```python
from build123d import *

# Parameters (mm, degrees)
SKETCH_1_W          = 58.5
SKETCH_1_H          = 42
EXTRUDE_1_DEPTH     = 123
CUT_EXTRUDE_1_DEPTH = 120
SKETCH_3_W          = 52.5
SKETCH_3_H          = 3
CUT_EXTRUDE_2_DEPTH = 25
FILLET_1_R          = 3
SKETCH_4_W          = 7
SKETCH_4_H          = 123
EXTRUDE_2_DEPTH     = 3
HOLE_WIZARD_1_D     = 3.5
SKETCH_7_2_W        = 7
SKETCH_7_2_H        = 83
CUT_EXTRUDE_3_DEPTH = 3
SKETCH_9_W          = 52.5
SKETCH_9_H          = 36
EXTRUDE_3_DEPTH     = 10


with BuildPart() as part:
    # 草图1 → 凸台-拉伸1 (new body)
    with BuildSketch(Plane(origin=(0, 0, 0), x_dir=(1, 0, 0), z_dir=(0, 1, 0))):
        with Locations((29.25, 21)):
            Rectangle(SKETCH_1_W, SKETCH_1_H)
    extrude(amount=EXTRUDE_1_DEPTH)

    # 草图2 → 切除-拉伸1 (cut)
    with BuildSketch(Plane(origin=(0, 123, 0), x_dir=(1, 0, 0), z_dir=(0, 1, 0))):
        Polygon((3, 3), (4.178571429, 3), (54.321428571, 39), (3, 39), align=None)
        Polygon((54.321428571, 39), (4.178571429, 3), (55.5, 3), (55.5, 39), align=None)
    extrude(amount=-CUT_EXTRUDE_1_DEPTH, mode=Mode.SUBTRACT)

    # 草图3 → 切除-拉伸2 (cut)
    with BuildSketch(Plane(origin=(0, 123, 0), x_dir=(1, 0, 0), z_dir=(0, 1, 0))):
        with Locations((29.25, 1.5)):
            Rectangle(SKETCH_3_W, SKETCH_3_H)
    extrude(amount=-CUT_EXTRUDE_2_DEPTH, mode=Mode.SUBTRACT)

    # 圆角1
    fillet_1_edges = [part.edges().sort_by_distance(p)[0] for p in [
        (3, 98, -1.5),
        (55.5, 98, -1.5),
    ]]
    fillet(fillet_1_edges, radius=FILLET_1_R)

    # 草图4 → 凸台-拉伸2 (add)
    with BuildSketch(Plane(origin=(0, 0, -42), x_dir=(-1, 0, 0), z_dir=(0, 0, -1))):
        with Locations((-62, 61.5)):
            Rectangle(SKETCH_4_W, SKETCH_4_H)
        with Locations((3.5, 61.5)):
            Rectangle(SKETCH_4_W, SKETCH_4_H)
    extrude(amount=-EXTRUDE_2_DEPTH)

    # 孔1 (through all)
    with Locations(Plane(origin=(0, 0, -42), x_dir=(-1, 0, 0), z_dir=(0, 0, -1))):
        with Locations((-62, 3.5), (3.5, 3.5), (3.5, 119.5), (-62, 119.5)):
            Hole(HOLE_WIZARD_1_D / 2)

    # Sketch 7 2 → 切除-拉伸3 (cut)
    with BuildSketch(Plane(origin=(0, 0, -42), x_dir=(-1, 0, 0), z_dir=(0, 0, -1))):
        with Locations((3.5, 61.5)):
            Rectangle(SKETCH_7_2_W, SKETCH_7_2_H)
        with Locations((-62, 61.5)):
            Rectangle(SKETCH_7_2_W, SKETCH_7_2_H)
    extrude(amount=-CUT_EXTRUDE_3_DEPTH, mode=Mode.SUBTRACT)

    # 草图9 → 凸台-拉伸3 (add)
    with BuildSketch(Plane(origin=(0, 3, 0), x_dir=(1, 0, 0), z_dir=(0, 1, 0))):
        with Locations((29.25, 21)):
            Rectangle(SKETCH_9_W, SKETCH_9_H)
    extrude(amount=EXTRUDE_3_DEPTH)


solid = part.part
```
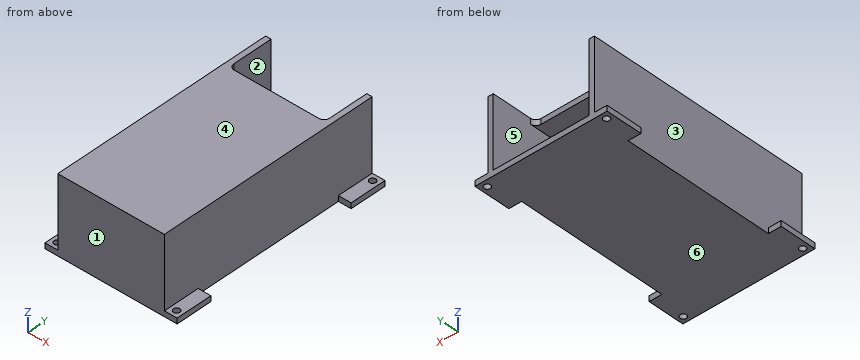
CAD build for the part. Positions are in the model's coordinates, mm. Face numbers are marked on the shaded views. A direction names the side the tool comes from. Give positions to 0.01 mm unless a question says otherwise; leave off trailing zeros. Loops run counter-clockwise (first coordinate to the right, second up) from the corner with the lowest first, then second, coordinate; pieces in that order, holes last. Notation, with made-up numbers: (88.25, 45) - (137.25, 45) arc R19 cw to (137.25, 65) - close; hole circle Ø6 at (30.25, 47). An arc over 180 degrees is marked (long way). Put each result on its own line as item: value.
Q1. Mould opens along Z. For the marked faces 3, 4, 5 and 6 say: pulls with the +Z half, pulls with the -Z half, needs draft (parallel to the pull), parting line crosses it, or undercut.
Filled in:
face 3: needs draft
face 4: pulls with the +Z half
face 5: undercut
face 6: pulls with the -Z half
Q2. Slice it at C-C (y = 60.5). Give the cut face in (x, z).
Filled in:
outline: (0, -42) - (58.5, -42) - (58.5, 0) - (0, 0) - close; hole (3, -39) - (55.5, -39) - (55.5, -3) - (3, -3) - close
Q3. Slice it at D-D (z = -14). Give the cut face in (x, y).
Filled in:
outline: (0, 0) - (58.5, 0) - (58.5, 123) - (55.5, 123) - (55.5, 13) - (3, 13) - (3, 123) - (0, 123) - close
Q4. Slice it at A-A (x = -3.5). Give the cut face in (y, z).
Filled in:
outline: (0, -42) - (1.75, -42) - (1.75, -39) - (0, -39) - close; (5.25, -42) - (20, -42) - (20, -39) - (5.25, -39) - close; (103, -42) - (117.75, -42) - (117.75, -39) - (103, -39) - close; (121.25, -42) - (123, -42) - (123, -39) - (121.25, -39) - close
Q5. Flat gauge pins, fed straight in: pin 1 (18 mm diameter, centred on x = 32, z = -19, fed in from +Y); pin 2 (1.5 mm diameter, centred on y = 69.5, z = -19.5, fed in from -X); pin 3 (11.5 mm diameter, centred on y = 70, z = -13, fed in from +X). Where does each tip first touch, or does it go through?
Filled in:
pin 1: stops at y = 13
pin 2: stops at x = 0
pin 3: stops at x = 58.5
Q6. Probe line 1 along Y through (x, z) = (62, -40.2); line 2 along Z through (x, y) = (37, 58.5); line 3 along X through (y, z) = (101, -4). List the from-to ranges inside material, lowest first.
Filled in:
line 1: y = 0 to 1.75, 5.25 to 20, 103 to 117.75, 121.25 to 123
line 2: z = -42 to -39, -3 to 0
line 3: x = 0 to 3, 55.5 to 58.5
Q7. Slice it at B-B (y = 119.5). Give the cut face in (x, z).
Filled in:
outline: (-7, -42) - (-5.25, -42) - (-5.25, -39) - (-7, -39) - close; (-1.75, -42) - (60.25, -42) - (60.25, -39) - (58.5, -39) - (58.5, 0) - (55.5, 0) - (55.5, -39) - (3, -39) - (3, 0) - (0, 0) - (0, -39) - (-1.75, -39) - close; (63.75, -42) - (65.5, -42) - (65.5, -39) - (63.75, -39) - close
Q8. Tool access for the marked faces 1 and 2: list every direction of +Z, -Z, +X, -X, +Y, -Y with a clear straight run to the whole face (end or side of a thin tool).
Filled in:
face 1: +Z, -Z, +X, -X, -Y
face 2: +Y
